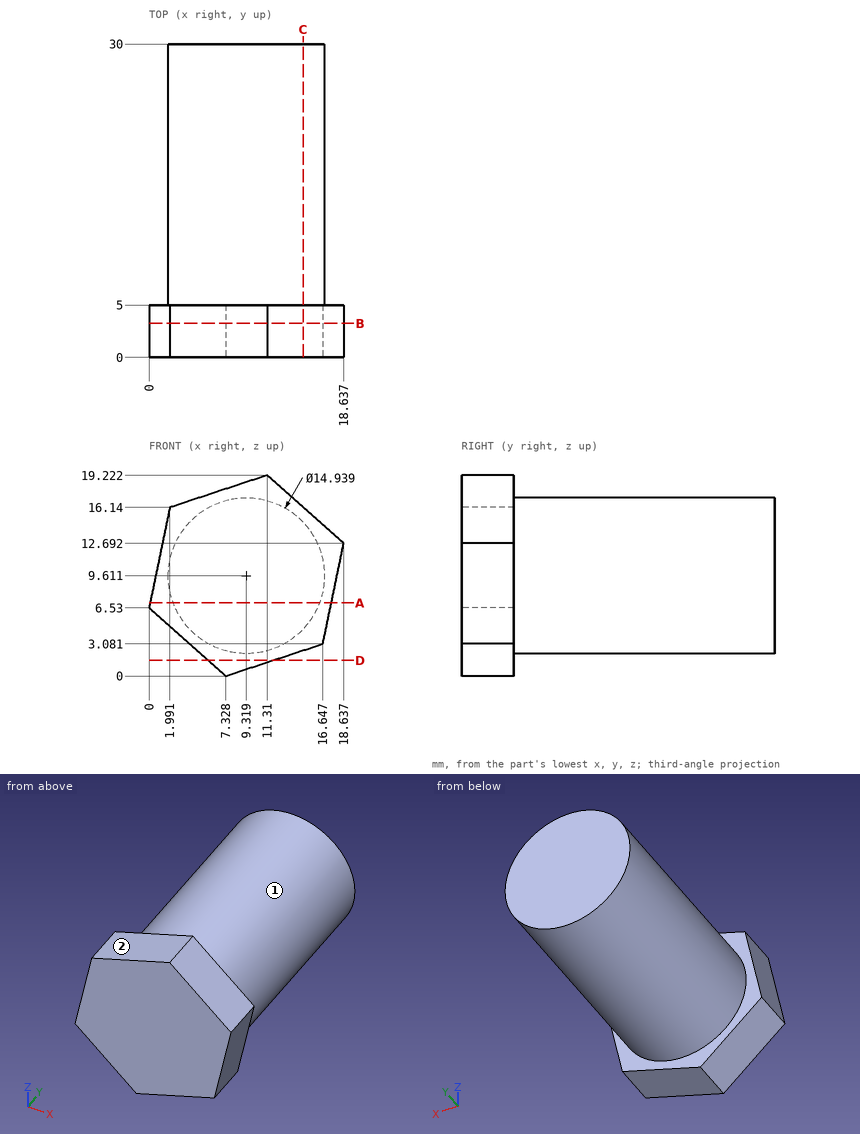
Could you check a few things on this drawing? It's one solid part, dimensions in mm from its lowest x, y, z. A direction names the side the tool comes from. Coordinates: 2 decimals unless noted, no trailing zeros. Write each loop counter-clockwise with the first axis right and the second up, starting at its lowest first coordinate (ties: lowest second). Pieces come first, ordered by that corner, then holes. Notation, with made-up numbers: M 59,45.25 L 104,45.25 A24 cw 104,73.25 Z; hole C -29,28.25 d9. An arc over 180 degrees is marked long. Answer as CSV lines item,"result". Start each with the question number.
Q1. Will these pins go through, and if not, where does the flat tip stop? pin 1 Ø3 at (y, z) = (18, 9) entering from +X; pin 2 Ø4 at (x, y) = (15, 25.5) entering from +Z; pin 3 Ø4 at (x, y) = (10.5, 12.5) entering from +Z.
Q2. Suppose I cut it at B-B, the plane y = 3.25. List the corners of the cut face in (x, z) for me, then the cut area to 3 significant figures.
Q3. Suppose I cut it at D-D, the plane z = 1.5. List the corners of the cut face in (x, y) for me (1 decimal), then the cut area to 3 significant figures.
Q4. I need wall thicknesses on probe 1 along Y at (x, z) = (16.5, 14.25); probe 2 along Z at (x, y) = (9.5, 5.5); probe 3 along Z at (x, y) = (11, 11.75). Which ranges of each line are inside material? Lowest first, please. Write a range as [from, to].
Q5. Suppose I cut it at C-C, the plane x = 14.75. List the corners of the cut face in (y, z) for me (1 decimal).
Q6. For the marked faces 1 and 2, which set-ups out of +Z, -Z, +X, -X, +Y, -Y let a thin tool reach every point of the face, with its end or its side?
Q7. Suppose I cut it at A-A, the plane z = 7. List the corners of the cut face in (x, y) for me, then the cut area to 3 significant figures.
Entries:
1,pin 1,"stops at x = 16.79"
1,pin 2,"stops at z = 16.11"
1,pin 3,"stops at z = 17.08"
2,outline,"M 0,6.53 L 7.33,0 L 16.65,3.08 L 18.64,12.69 L 11.31,19.22 L 1.99,16.14 Z"
2,area,"250 mm²"
3,outline,"M 5.6,0 L 11.9,0 L 11.9,5 L 5.6,5 Z"
3,area,"31.1 mm²"
4,probe 1,"y = [0, 5]"
4,probe 2,"z = [2.14, 17.08]"
4,probe 3,"z = [2.33, 16.89]"
5,outline,"M 0,2.5 L 5,2.5 L 5,4.5 L 30,4.5 L 30,14.7 L 5,14.7 L 5,16.2 L 0,16.2 Z"
6,face 1,"+Y"
6,face 2,"+Z, -X, +Y, -Y"
7,outline,"M 0.1,0 L 17.46,0 L 17.46,5 L 16.32,5 L 16.32,30 L 2.32,30 L 2.32,5 L 0.1,5 Z"
7,area,"437 mm²"
